from build123d import *

# Parameters (mm, degrees)
F0_W     = 46
F0_H     = 3
F0_W_2   = 50
F0_W_3   = 3
F0_H_2   = 20
F0_W_4   = 54
F1_DEPTH = 3


with BuildPart() as f1:
    # F0 (on Top) → F1 (new body)
    with BuildSketch(Plane.XY):
        with Locations((-227, 1.5)):
            Rectangle(F0_W, F0_H)
        Polygon((-204, 0), (-250, 0), (-250, -30), (-250, -50), (-250, -70), (-250, -90), (-250, -110), (0, -110), (0, -90), (0, -70), (0, -50), (0, -30), (0, 0), (-54, 0), (-104, 0), (-154, 0), align=None)
        with Locations((-178, -57.5)):
            Rectangle(F0_W_2, F0_H, mode=Mode.SUBTRACT)
        with Locations((-74.99309, -57.5)):
            Rectangle(F0_W_2, F0_H, mode=Mode.SUBTRACT)
        Polygon((-250, -30), (-250, 0), (-250, 3), (-253, 3), (-253, -30), align=None)
        with Locations((-129, 1.5)):
            Rectangle(F0_W_2, F0_H)
        with Locations((-251.5, -60)):
            Rectangle(F0_W_3, F0_H_2)
        with Locations((-27, 1.5)):
            Rectangle(F0_W_4, F0_H)
        with Locations((-251.5, -100)):
            Rectangle(F0_W_3, F0_H_2)
        Polygon((0, 3), (0, 0), (0, -30), (3, -30), (3, 3), align=None)
        with Locations((1.5, -100)):
            Rectangle(F0_W_3, F0_H_2)
        with Locations((1.5, -60)):
            Rectangle(F0_W_3, F0_H_2)
    extrude(amount=F1_DEPTH)


solid = f1.part
The model under review builds one solid part; all positions refer to its coordinate system, in mm. Coordinates: 2 decimals unless noted, no trailing zeros. Loops run counter-clockwise (first coordinate to the right, second up) from the corner with the lowest first, then second, coordinate; pieces in that order, holes last. Notation, with made-up numbers: (58.25, -4.75) -> (80.25, -4.75) arc R29 ccw to (80.25, 29.25) -> close; hole circle Ø5 at (44, -16.5). An arc over 180 degrees is marked (long way). Use a Markdown table: item, result. Add a question column.
1. Add section C-C on y = -82. Write out the cut boundary in (x, z), plus the area to 3 significant figures.
2. Add section A-A on x = -68.5. Write out the cut boundary in (y, z).
3. Add section B-B on z = 1.5. Give the number of separate pieces and of enclosed holes in the cut face, plus the area to 3 significant figures.
4. To check wall thickness, follow line 1 (Y direction, x = -80, z = 0.55); line 2 (X direction, y = -33.5, z = 0.4). State the ranges of each line that lie inside material, in increasing order.
5. Clearance check with flat-ended pins moving along their axes: pin 1 Ø1 at (x, y) = (-95, -38) entering from -Z; pin 2 Ø0.9 at (x, z) = (-73, 1) entering from +Y; pin 3 Ø0.9 at (y, z) = (-81, 1) entering from +X. State where each tip first meets the part, or that it passes through.
Returned:
| question | item | result |
|---|---|---|
| 1 | outline | (-250, 0) -> (0, 0) -> (0, 3) -> (-250, 3) -> close |
| 1 | area | 750 mm² |
| 2 | outline | (-110, 0) -> (-59, 0) -> (-59, 3) -> (-110, 3) -> close; (-56, 0) -> (0, 0) -> (0, 3) -> (-56, 3) -> close |
| 3 | separate pieces | 1 |
| 3 | enclosed holes | 2 |
| 3 | area | 28,100 mm² |
| 4 | line 1 | y = -110 to -59, -56 to 0 |
| 4 | line 2 | x = -250 to 0 |
| 5 | pin 1 | stops at z = 0 |
| 5 | pin 2 | stops at y = 0 |
| 5 | pin 3 | stops at x = 0 |
